```python
from build123d import *

# Parameters (mm, degrees)
SKIZZE1_R                            = 26.5
SKIZZE1_R_2                          = 25
AUFSATZ_LINEAR_AUSTRAGEN1_DEPTH      = 90
SCHNITT_LINEAR_AUSTRAGEN1_DEPTH      = 98.491025228
SCHNITT_LINEAR_AUSTRAGEN1_DEPTH_BACK = 98.491025228
SKIZZE2_W                            = 47.420755097
SKIZZE2_H                            = 0.5
AUFSATZ_LINEAR_AUSTRAGEN2_DEPTH      = 47.420755097
AUFSATZ_LINEAR_AUSTRAGEN3_DEPTH      = 2.25
AUFSATZ_LINEAR_AUSTRAGEN3_DEPTH_BACK = 2.25
SCHNITT_LINEAR_AUSTRAGEN2_DEPTH      = 30
AUFSATZ_LINEAR_AUSTRAGEN4_DEPTH      = 30
AUFSATZ_LINEAR_AUSTRAGEN5_DEPTH      = 1
SPIEGELN2_COPY_1_DEPTH               = 30
SPIEGELN2_COPY_2_DEPTH               = 30
SPIEGELN2_COPY_3_DEPTH               = 1
SCHNITT_LINEAR_AUSTRAGEN3_DEPTH      = 2.25
SCHNITT_LINEAR_AUSTRAGEN3_DEPTH_BACK = 2.25


with BuildPart() as part:
    # Skizze1 → Aufsatz-Linear austragen1 (new body)
    with BuildSketch(Plane.XY):
        with Locations(Location((0, 0, 0), (0, 0, 180))):
            Circle(SKIZZE1_R)
        with Locations(Location((0, 0, 0), (0, 0, 180))):
            Circle(SKIZZE1_R_2, mode=Mode.SUBTRACT)
    extrude(amount=AUFSATZ_LINEAR_AUSTRAGEN1_DEPTH)

    # Skizze2 → Schnitt-Linear austragen1 (cut, two sides: drawn at the far end of the back side and taken through both)
    with BuildSketch(Plane(origin=(0, 0, 0), x_dir=(0, 0, -1), z_dir=(1, 0, 0)).offset(-SCHNITT_LINEAR_AUSTRAGEN1_DEPTH_BACK)):
        with Locations((-23.710377549, 26.25)):
            Rectangle(SKIZZE2_W, SKIZZE2_H)
    extrude(amount=SCHNITT_LINEAR_AUSTRAGEN1_DEPTH + SCHNITT_LINEAR_AUSTRAGEN1_DEPTH_BACK, mode=Mode.SUBTRACT)

    # Skizze4 → Aufsatz-Linear austragen2 (add)
    with BuildSketch(Plane(origin=(0, 0, 0), x_dir=(-1, 0, 0), z_dir=(0, 0, -1))):
        Polygon((8.529361055, 23.5), (-8.529361055, 23.5), (-5.360314204, 25.204344352), (5.360314204, 25.204344352), align=None)
    extrude(amount=-AUFSATZ_LINEAR_AUSTRAGEN2_DEPTH)

    # Skizze5 → Aufsatz-Linear austragen3 (add, two sides: drawn at the far end of the back side and taken through both)
    with BuildSketch(Plane(origin=(0, 0, 0), x_dir=(0, 0, -1), z_dir=(1, 0, 0)).offset(-AUFSATZ_LINEAR_AUSTRAGEN3_DEPTH_BACK)):
        Polygon((-12.029982204, 26), (-11.783333845, 26), (-11.783333845, 26.449227107), (-13.320755097, 26.449227107), (-13.769982204, 26), (-12.871527991, 26), align=None)
        Polygon((-41.420755097, 26), (-38.971527991, 26), (-39.420755097, 26.449227107), (-41.420755097, 26.449227107), align=None)
        Polygon((-38.129982204, 26), (-37.231527991, 26), (-37.680755097, 26.449227107), align=None)
        Polygon((-36.389982204, 26), (-35.491527991, 26), (-35.940755097, 26.449227107), align=None)
        Polygon((-34.649982204, 26), (-33.751527991, 26), (-34.200755097, 26.449227107), align=None)
        Polygon((-32.909982204, 26), (-32.011527991, 26), (-32.460755097, 26.449227107), align=None)
        Polygon((-31.169982204, 26), (-30.271527991, 26), (-30.720755097, 26.449227107), align=None)
        Polygon((-29.429982204, 26), (-28.531527991, 26), (-28.980755097, 26.449227107), align=None)
        Polygon((-27.689982204, 26), (-26.791527991, 26), (-27.240755097, 26.449227107), align=None)
        Polygon((-25.949982204, 26), (-25.051527991, 26), (-25.500755097, 26.449227107), align=None)
        Polygon((-24.209982204, 26), (-23.311527991, 26), (-23.760755097, 26.449227107), align=None)
        Polygon((-22.469982204, 26), (-21.571527991, 26), (-22.020755097, 26.449227107), align=None)
        Polygon((-20.729982204, 26), (-19.831527991, 26), (-20.280755097, 26.449227107), align=None)
        Polygon((-18.989982204, 26), (-18.091527991, 26), (-18.540755097, 26.449227107), align=None)
        Polygon((-17.249982204, 26), (-16.351527991, 26), (-16.800755097, 26.449227107), align=None)
        Polygon((-15.509982204, 26), (-14.611527991, 26), (-15.060755097, 26.449227107), align=None)
    extrude(amount=AUFSATZ_LINEAR_AUSTRAGEN3_DEPTH + AUFSATZ_LINEAR_AUSTRAGEN3_DEPTH_BACK)

    # Skizze6 → Schnitt-Linear austragen2 (cut)
    with BuildSketch(Plane(origin=(0, 0, 0), x_dir=(-1, 0, 0), z_dir=(0, 0, -1))):
        with BuildLine():
            Line((-16.716780274, 19.403786042), (-17.346601449, 20.033607218))
            ThreePointArc((-17.346601449, 20.033607218), (-18.738329701, 18.738329701), (-20.033607218, 17.346601449))
            Line((-20.033607218, 17.346601449), (-19.403786042, 16.716780274))
            Line((-19.403786042, 16.716780274), (-18.97004537, 16.283039601))
            ThreePointArc((-18.97004537, 16.283039601), (-17.67766953, 17.67766953), (-16.283039601, 18.97004537))
            Line((-16.283039601, 18.97004537), (-16.716780274, 19.403786042))
        make_face()
        with BuildLine():
            Line((-17.346601449, 20.033607218), (-17.394826817, 20.081832586))
            Line((-17.394826817, 20.081832586), (-18.854928678, 18.854928678))
            Line((-18.854928678, 18.854928678), (-20.081832586, 17.394826817))
            Line((-20.081832586, 17.394826817), (-20.033607218, 17.346601449))
            ThreePointArc((-20.033607218, 17.346601449), (-18.738329701, 18.738329701), (-17.346601449, 20.033607218))
        make_face()
        with BuildLine():
            Line((-15.273506474, 17.960512242), (-16.283039601, 18.97004537))
            ThreePointArc((-16.283039601, 18.97004537), (-17.67766953, 17.67766953), (-18.97004537, 16.283039601))
            Line((-18.97004537, 16.283039601), (-17.960512242, 15.273506474))
            Line((-17.960512242, 15.273506474), (-15.273506474, 17.960512242))
        make_face()
    schnitt_linear_austragen2 = extrude(amount=-SCHNITT_LINEAR_AUSTRAGEN2_DEPTH, mode=Mode.SUBTRACT)

    # Skizze6<3> → Aufsatz-Linear austragen4 (add)
    with BuildSketch(Plane(origin=(0, 0, 0), x_dir=(-1, 0, 0), z_dir=(0, 0, -1))):
        with BuildLine():
            ThreePointArc((-15.109260367, 19.917586479), (-15.703298471, 19.452671208), (-16.283039601, 18.97004537))
            Line((-16.283039601, 18.97004537), (-15.273506474, 17.960512242))
            Line((-15.273506474, 17.960512242), (-17.960512242, 15.273506474))
            Line((-17.960512242, 15.273506474), (-18.97004537, 16.283039601))
            ThreePointArc((-18.97004537, 16.283039601), (-19.452671208, 15.703298471), (-19.917586479, 15.109260367))
            Line((-19.917586479, 15.109260367), (-17.960512242, 13.15218613))
            Line((-17.960512242, 13.15218613), (-13.15218613, 17.960512242))
            Line((-13.15218613, 17.960512242), (-15.109260367, 19.917586479))
        make_face()
    aufsatz_linear_austragen4 = extrude(amount=-AUFSATZ_LINEAR_AUSTRAGEN4_DEPTH)

    # Skizze7 → Aufsatz-Linear austragen5 (add)
    with BuildSketch(Plane.XY.offset(30)):
        Polygon((13.15218613, 17.960512242), (17.960512242, 13.15218613), (19.917586479, 15.109260367), (18.25472482, 18.000193095), (15.352274142, 20.160600254), align=None)
    aufsatz_linear_austragen5 = extrude(amount=AUFSATZ_LINEAR_AUSTRAGEN5_DEPTH)

    # Spiegeln1: Schnitt-Linear austragen2, Aufsatz-Linear austragen4, Aufsatz-Linear austragen5 across plane
    add(schnitt_linear_austragen2.mirror(Plane(origin=(0, 0, 0), x_dir=(0, 0, 1), z_dir=(1, 0, 0))), mode=Mode.SUBTRACT)
    add(aufsatz_linear_austragen4.mirror(Plane(origin=(0, 0, 0), x_dir=(0, 0, 1), z_dir=(1, 0, 0))))
    add(aufsatz_linear_austragen5.mirror(Plane(origin=(0, 0, 0), x_dir=(0, 0, 1), z_dir=(1, 0, 0))))

    # Spiegeln2: Schnitt-Linear austragen2, Aufsatz-Linear austragen4, Aufsatz-Linear austragen5 across plane
    add(schnitt_linear_austragen2.mirror(Plane.ZX), mode=Mode.SUBTRACT)
    add(aufsatz_linear_austragen4.mirror(Plane.ZX))
    add(aufsatz_linear_austragen5.mirror(Plane.ZX))

    # Spiegeln2 copy 1 sketch → Spiegeln2 copy 1 (cut)
    with BuildSketch(Plane(origin=(0, 0, 0), x_dir=(1, 0, 0), z_dir=(0, 0, -1))):
        with BuildLine():
            Line((-16.716780274, 19.403786042), (-17.346601449, 20.033607218))
            ThreePointArc((-17.346601449, 20.033607218), (-18.738329701, 18.738329701), (-20.033607218, 17.346601449))
            Line((-20.033607218, 17.346601449), (-19.403786042, 16.716780274))
            Line((-19.403786042, 16.716780274), (-18.97004537, 16.283039601))
            ThreePointArc((-18.97004537, 16.283039601), (-17.67766953, 17.67766953), (-16.283039601, 18.97004537))
            Line((-16.283039601, 18.97004537), (-16.716780274, 19.403786042))
        make_face()
        with BuildLine():
            Line((-17.346601449, 20.033607218), (-17.394826817, 20.081832586))
            Line((-17.394826817, 20.081832586), (-18.854928678, 18.854928678))
            Line((-18.854928678, 18.854928678), (-20.081832586, 17.394826817))
            Line((-20.081832586, 17.394826817), (-20.033607218, 17.346601449))
            ThreePointArc((-20.033607218, 17.346601449), (-18.738329701, 18.738329701), (-17.346601449, 20.033607218))
        make_face()
        with BuildLine():
            Line((-15.273506474, 17.960512242), (-16.283039601, 18.97004537))
            ThreePointArc((-16.283039601, 18.97004537), (-17.67766953, 17.67766953), (-18.97004537, 16.283039601))
            Line((-18.97004537, 16.283039601), (-17.960512242, 15.273506474))
            Line((-17.960512242, 15.273506474), (-15.273506474, 17.960512242))
        make_face()
    extrude(amount=-SPIEGELN2_COPY_1_DEPTH, mode=Mode.SUBTRACT)

    # Spiegeln2 copy 2 sketch → Spiegeln2 copy 2 (add)
    with BuildSketch(Plane(origin=(0, 0, 0), x_dir=(1, 0, 0), z_dir=(0, 0, -1))):
        with BuildLine():
            ThreePointArc((-15.109260367, 19.917586479), (-15.703298471, 19.452671208), (-16.283039601, 18.97004537))
            Line((-16.283039601, 18.97004537), (-15.273506474, 17.960512242))
            Line((-15.273506474, 17.960512242), (-17.960512242, 15.273506474))
            Line((-17.960512242, 15.273506474), (-18.97004537, 16.283039601))
            ThreePointArc((-18.97004537, 16.283039601), (-19.452671208, 15.703298471), (-19.917586479, 15.109260367))
            Line((-19.917586479, 15.109260367), (-17.960512242, 13.15218613))
            Line((-17.960512242, 13.15218613), (-13.15218613, 17.960512242))
            Line((-13.15218613, 17.960512242), (-15.109260367, 19.917586479))
        make_face()
    extrude(amount=-SPIEGELN2_COPY_2_DEPTH)

    # Spiegeln2 copy 3 sketch → Spiegeln2 copy 3 (add)
    with BuildSketch(Plane(origin=(0, 0, 30), x_dir=(-1, 0, 0), z_dir=(0, 0, 1))):
        Polygon((13.15218613, 17.960512242), (17.960512242, 13.15218613), (19.917586479, 15.109260367), (18.25472482, 18.000193095), (15.352274142, 20.160600254), align=None)
    extrude(amount=SPIEGELN2_COPY_3_DEPTH)

    # Skizze5<3> → Schnitt-Linear austragen3 (cut, two sides: drawn at the far end of the back side and taken through both)
    with BuildSketch(Plane(origin=(0, 0, 0), x_dir=(0, 0, -1), z_dir=(1, 0, 0)).offset(-SCHNITT_LINEAR_AUSTRAGEN3_DEPTH_BACK)):
        Polygon((-38.550755097, 25.579227107), (-38.129982204, 26), (-38.971527991, 26), align=None)
        Polygon((-36.810755097, 25.579227107), (-36.389982204, 26), (-37.231527991, 26), align=None)
        Polygon((-35.070755097, 25.579227107), (-34.649982204, 26), (-35.491527991, 26), align=None)
        Polygon((-33.330755097, 25.579227107), (-32.909982204, 26), (-33.751527991, 26), align=None)
        Polygon((-31.590755097, 25.579227107), (-31.169982204, 26), (-32.011527991, 26), align=None)
        Polygon((-29.850755097, 25.579227107), (-29.429982204, 26), (-30.271527991, 26), align=None)
        Polygon((-28.110755097, 25.579227107), (-27.689982204, 26), (-28.531527991, 26), align=None)
        Polygon((-26.370755097, 25.579227107), (-25.949982204, 26), (-26.791527991, 26), align=None)
        Polygon((-24.630755097, 25.579227107), (-24.209982204, 26), (-25.051527991, 26), align=None)
        Polygon((-22.890755097, 25.579227107), (-22.469982204, 26), (-23.311527991, 26), align=None)
        Polygon((-21.150755097, 25.579227107), (-20.729982204, 26), (-21.571527991, 26), align=None)
        Polygon((-19.385368651, 25.604613553), (-18.989982204, 26), (-19.831527991, 26), (-19.410755097, 25.579227107), align=None)
        Polygon((-17.645368651, 25.604613553), (-17.249982204, 26), (-18.091527991, 26), (-17.696141544, 25.604613553), (-17.670755097, 25.579227107), align=None)
        Polygon((-15.535368651, 25.974613553), (-15.509982204, 26), (-16.351527991, 26), (-16.326141544, 25.974613553), (-15.930755097, 25.579227107), align=None)
        Polygon((-13.795368651, 25.974613553), (-13.769982204, 26), (-14.611527991, 26), (-14.586141544, 25.974613553), (-14.190755097, 25.579227107), align=None)
    extrude(amount=SCHNITT_LINEAR_AUSTRAGEN3_DEPTH + SCHNITT_LINEAR_AUSTRAGEN3_DEPTH_BACK, mode=Mode.SUBTRACT)


solid = part.part
```
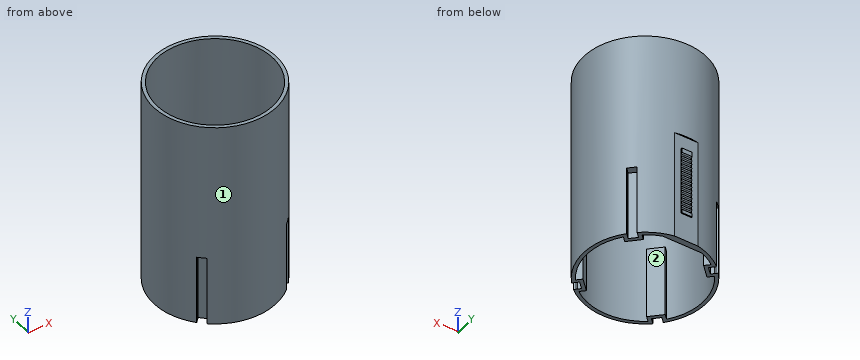
Here's how the part is built. I have some questions about the finished solid (model axes, mm). Face numbers are marked on the shaded views. Round coordinates to 2 decimals unless told otherwise and drop trailing zeros. Loops run counter-clockwise (first coordinate to the right, second up) from the corner with the lowest first, then second, coordinate; pieces in that order, holes last.
1. If I drill on probe 1 along Y at (x, z) = (0, 49); probe 2 along X at (y, z) = (16, 20.5); probe 3 along Y at (x, z) = (20, 59), over which ranges is the centre line in solid material (lowest first)?
Answers:
probe 1: y = -26.5 to -25, 25 to 26.5
probe 2: x = -21.12 to -18.69, -17.23 to -15.11, 15.11 to 17.23, 18.69 to 21.12
probe 3: y = -17.39 to -15, 15 to 17.39
2. Thinking about a two-plate mould opening in Y: for the marked faces 1 and 2, which applies, released by +Y, released by -Y, zero draft, split by the parting line, or undercut?
Answers:
face 1: split by the parting line
face 2: undercut
3. Suppose I cut it at A-A, the plane y = 0. Please give me the cut outline in (x, z), and give its area (3 significant figures).
Answers:
outline: (-26.5, 0) - (-25, 0) - (-25, 90) - (-26.5, 90) - close; (25, 0) - (26.5, 0) - (26.5, 90) - (25, 90) - close
area: 270 mm2
4. Suppose I cut it at D-D, the plane y = 8.5. Please give me the cut outline in (x, z).
Answers:
outline: (-25.1, 0) - (-23.51, 0) - (-23.51, 90) - (-25.1, 90) - close; (23.51, 0) - (25.1, 0) - (25.1, 90) - (23.51, 90) - close
5. Suppose I cut it at B-B, the plane z = 80. Please give me the cut outline in (x, y), and give its area (3 significant figures).
Answers:
outline: circle Ø53 at (0, 0); hole circle Ø50 at (0, 0)
area: 243 mm2
6. Will these pins go through, and if not, where does the flat tip stop? pin 1 (12 mm diameter, centred on x = 3.5, z = 30, fed in from +Y); pin 2 (12 mm diameter, centred on x = -17, z = 50.5, fed in from -Y); pin 3 (8 mm diameter, centred on y = 6, z = 37, fed in from -X).
Answers:
pin 1: stops at y = 26.45
pin 2: stops at y = -24.11
pin 3: stops at x = -26.42
7. Suppose I cut it at C-C, the plane x = 4. Please give me the cut outline in (y, z).
Answers:
outline: (-26.2, 0) - (-24.68, 0) - (-24.68, 90) - (-26.2, 90) - close; (23.5, 0) - (26, 0) - (26, 47.42) - (26.2, 47.42) - (26.2, 90) - (24.68, 90) - (24.68, 47.42) - (23.5, 47.42) - close
